Source: CAD feature listing. Evaluate the final solid. Frame: model axes, mm. Give positions to 0.01 mm unless a question says otherwise; leave off trailing zeros. Order: outer loops, then holes, each group sorted by start corner. A loop starts at its lowest first (then second) coordinate and runs counter-clockwise, first axis right, second up. Notation, with made-up numbers: (82, 86) - (95, 86) arc R11 ccw to (95, 91) - close; hole circle Ø4 at (63.5, -10). An arc over 180 degrees is marked (long way). One line per item, written item: value. Start each with the question number.
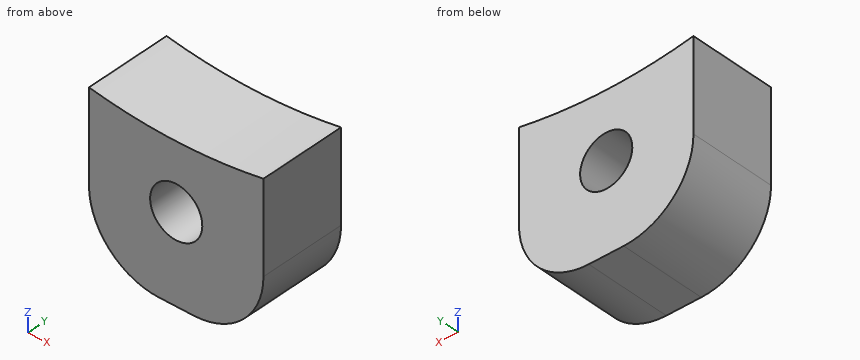
from build123d import *

# Parameters (mm, degrees)
EXTRUDE1_DEPTH            = 6.35
SKETCH2_R                 = 36.5125
CUT_EXTRUDE1_DEPTH        = 6.35
F_6_CLEARANCE_HOLE1_D     = 3.7973
F_6_CLEARANCE_HOLE1_DEPTH = 330.2
F_6_CLEARANCE_HOLE1_TIP   = 1.140824014


with BuildPart() as part:
    # Sketch1 → Extrude1 (new body)
    with BuildSketch(Plane(origin=(0, 0, 0), x_dir=(1, 0, 0), z_dir=(0, 1, 0))):
        with BuildLine():
            Line((-1.27, 22.225), (1.27, 22.225))
            ThreePointArc((1.27, 22.225), (4.862102448, 20.737102448), (6.35, 17.145))
            Line((6.35, 17.145), (6.35, -25.4))
            Line((6.35, -25.4), (-6.35, -25.4))
            Line((-6.35, -25.4), (-6.35, 17.145))
            ThreePointArc((-6.35, 17.145), (-4.862102448, 20.737102448), (-1.27, 22.225))
        make_face()
    extrude(amount=EXTRUDE1_DEPTH)

    # Sketch2 → Cut-Extrude1 (cut)
    with BuildSketch(Plane(origin=(0, 6.35, 0), x_dir=(-1, 0, 0), z_dir=(0, 1, 0))):
        with Locations((0, 25.4)):
            Circle(SKETCH2_R)
    extrude(amount=-CUT_EXTRUDE1_DEPTH, mode=Mode.SUBTRACT)

    # #6 Clearance Hole1
    with Locations(Plane(origin=(0, 6.35, -15.875), x_dir=(0, 0, 1), z_dir=(0, 1, 0))):
        with Locations((0, 0)):
            Hole(F_6_CLEARANCE_HOLE1_D / 2, depth=F_6_CLEARANCE_HOLE1_DEPTH)
            with Locations((0, 0, -(F_6_CLEARANCE_HOLE1_DEPTH + F_6_CLEARANCE_HOLE1_TIP / 2))):  # 118° drill point
                Cone(0, F_6_CLEARANCE_HOLE1_D / 2, F_6_CLEARANCE_HOLE1_TIP, mode=Mode.SUBTRACT)


solid = part.part
1. Contact query for flat-ended pins moving along their axis: pin 1 Ø1.5 at (x, y) = (4.5, 5.5) entering from +Z; pin 2 Ø2.5 at (x, z) = (0, -15.875) entering from -Y; pin 3 Ø1.5 at (x, y) = (-2, 1.5) entering from +Z; pin 4 Ø1 at (x, y) = (-2, 1.5) entering from -Z. Output: stop coordinate, or through.
2. Ray query, L1, parallel to Z at x = 1.5, y = 0.75; L2, parallel to X at y = 2, z = -16.5; L3, parallel to X at y = 2.5, z = -16.75 (3 decimals). Return the intervals inside material, ascending.
3. Section C-C on z = -16.5. Return the cut outline in (x, y), then the cut area to 3 significant figures.
4. Section D-D on z = -18.75. Return the cut outline in (x, y), then the cut area to 3 significant figures.
Data:
1. pin 1: stops at z = -10.73
1. pin 2: passes through
1. pin 3: stops at z = -11.01
1. pin 4: stops at z = -22.22
2. L1: z = -22.22 to -17.04, -14.71 to -11.08
2. L2: x = -6.35 to -1.79, 1.79 to 6.35
2. L3: x = -6.35 to -1.685, 1.685 to 6.35
3. outline: (-6.35, 0) - (-1.79, 0) - (-1.79, 6.35) - (-6.35, 6.35) - close; (1.79, 0) - (6.35, 0) - (6.35, 6.35) - (1.79, 6.35) - close
3. area: 57.9 mm2
4. outline: (-6.09, 0) - (6.09, 0) - (6.09, 6.35) - (-6.09, 6.35) - close
4. area: 77.3 mm2
